Source: CAD feature listing. Evaluate the final solid. Frame: model axes, mm. Face numbers are marked on the shaded views. A direction names the side the tool comes from. Coordinates: 2 decimals unless noted, no trailing zeros. Write each loop counter-clockwise with the first axis right and the second up, starting at its lowest first coordinate (ties: lowest second). Pieces come first, ordered by that corner, then holes. Notation, with made-up numbers: (12.5, 34.25) - (54.5, 34.25) arc R13 cw to (54.5, 56.25) - close; hole circle Ø2 at (40.25, 76.25). An arc over 180 degrees is marked (long way). One line per item, written item: value.
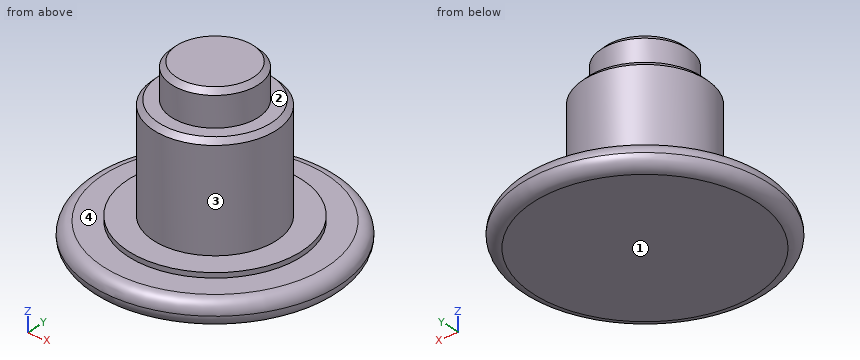
from build123d import *

# Parameters (mm, degrees)
F0_R     = 4.95
F1_DEPTH = 8.5
F2_R     = 7
F3_DEPTH = 0.4
F4_R     = 10
F5_DEPTH = 2
F6_R     = 0.99999
F7_R     = 3.5
F8_DEPTH = 2.8
F9_SIZE  = 0.4


# Not quite as in the source:
# - a fillet or chamfer is up to 0.001 mm smaller than in the source, because OpenCascade refuses the exact size


with BuildPart() as f1:
    # F0 (on Top) → F1 (new body)
    with BuildSketch(Plane.XY):
        Circle(F0_R)
    extrude(amount=F1_DEPTH)

    # F2 (on Top) → F3 (join)
    with BuildSketch(Plane.XY):
        Circle(F2_R)
    extrude(amount=-F3_DEPTH)

    # F4 (on face) → F5 (join)
    with BuildSketch(Plane(origin=(0, 0, -0.4), x_dir=(1, 0, 0), z_dir=(0, 0, -1))):
        Circle(F4_R)
    extrude(amount=F5_DEPTH)

    # F6 (radius 1 in the source; OpenCascade refuses exactly that, so slightly less here)
    f6_edges = [f1.edges().sort_by_distance(p)[0] for p in [
        (-10, 0, -2.4),
        (-10, 0, -0.4),
    ]]
    fillet(f6_edges, radius=F6_R)

    # F7 (on face) → F8 (join)
    with BuildSketch(Plane.XY.offset(8.5)):
        Circle(F7_R)
    extrude(amount=F8_DEPTH)

    # F9
    f9_edges = [f1.edges().sort_by_distance(p)[0] for p in [
        (-3.5, 0, 11.3),
        (-4.95, 0, 8.5),
    ]]
    chamfer(f9_edges, length=F9_SIZE)


solid = f1.part
1) Section query C-C on z = 9.75. Output: boundary loops of the cut face in (x, y), then the cut area to 3 significant figures.
Values found:
outline: circle Ø7 at (0, 0)
area: 38.5 mm2
2) Draft query along Y for the marked faces 3 and 4. Return one class per face: released by +Y, released by -Y, zero draft, split by the parting line, or undercut.
Values found:
face 3: split by the parting line
face 4: zero draft
3) Section query D-D on z = 7.75. Output: boundary loops of the cut face in (x, y), then the cut area to 3 significant figures.
Values found:
outline: circle Ø9.9 at (0, 0)
area: 77.0 mm2
4) Contact query for flat-ended pins moving along their axis: P1, Ø3, axis at x = -5, y = -7, coming from the +Z side; P2, Ø6, axis at x = -6, y = 3, coming from the +Z side; P3, Ø5, axis at x = 7.5, y = -4, coming from the +Z side. Output: stop coordinate, or through.
Values found:
P1: z = -0.4
P2: z = 8.5
P3: z = 0
5) Material intervals for line 1 (Z direction, x = -6, y = 5.25); line 2 (Z direction, x = 3, y = -4.5); line 3 (Y direction, x = 2.75, z = 0.5), sorted ascending.
Values found:
line 1: -2.4 to -0.4
line 2: -2.4 to 0
line 3: -4.12 to 4.12
6) Reachability of the marked faces 1 and 2 from +Z, -Z, +X, -X, +Y, -Y: full face, straight path, thin tool, end or side. Return the list, or none.
Values found:
face 1: -Z, +X, -X, +Y, -Y
face 2: +Z
